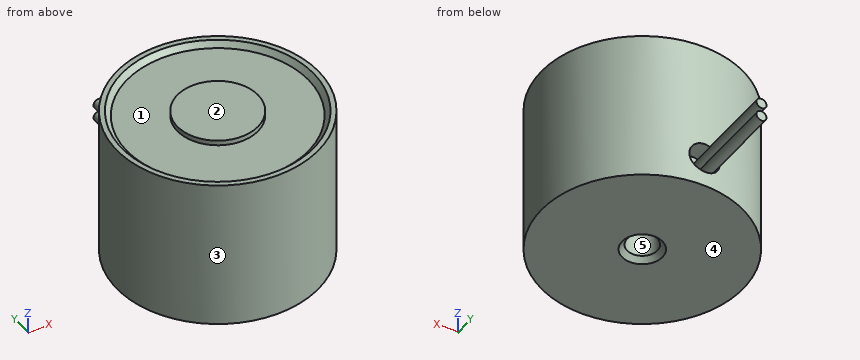
```python
from build123d import *

# Parameters (mm, degrees)
SKETCH_1_R          = 10
EXTRUDE_1_DEPTH     = 15
SKETCH_2_R          = 9
SKETCH_2_R_2        = 4
CUT_EXTRUDE_2_DEPTH = 0.5
CHAMFER_1_SIZE      = 0.5
SKETCH_3_R          = 1.5
CUT_EXTRUDE_3_DEPTH = 5
CHAMFER_2_SIZE      = 0.5
SKETCH_4_R          = 1.5
CUT_EXTRUDE_4_DEPTH = 7
SKETCH_5_R          = 0.5
EXTRUDE_2_DEPTH     = 10


with BuildPart() as part:
    # 草图1 → 凸台-拉伸1 (new body)
    with BuildSketch(Plane.XY):
        Circle(SKETCH_1_R)
    extrude(amount=EXTRUDE_1_DEPTH)

    # 草图2 → 切除-拉伸2 (cut)
    with BuildSketch(Plane.XY.offset(15)):
        Circle(SKETCH_2_R)
        Circle(SKETCH_2_R_2, mode=Mode.SUBTRACT)
    extrude(amount=-CUT_EXTRUDE_2_DEPTH, mode=Mode.SUBTRACT)

    # 倒角1
    chamfer_1_edges = [part.edges().sort_by_distance(p)[0] for p in [
        (-9, 0, 15),
    ]]
    chamfer(chamfer_1_edges, length=CHAMFER_1_SIZE - 0.0001)  # a hair under: the kernel refuses the full size

    # 草图3 → 切除-拉伸3 (cut)
    with BuildSketch(Plane(origin=(0, 0, 0), x_dir=(-1, 0, 0), z_dir=(0, 0, -1))):
        Circle(SKETCH_3_R)
    extrude(amount=-CUT_EXTRUDE_3_DEPTH, mode=Mode.SUBTRACT)

    # 倒角2
    chamfer_2_edges = [part.edges().sort_by_distance(p)[0] for p in [
        (1.5, 0, 0),
    ]]
    chamfer(chamfer_2_edges, length=CHAMFER_2_SIZE)

    # 草图4 → 切除-拉伸4 (cut)
    with BuildSketch(Plane(origin=(0, 8, 0), x_dir=(1, 0, 0), z_dir=(0, 1, 0))):
        with Locations(Location((0, -3, 0), (0, 0, 90))):
            Circle(SKETCH_4_R)
    extrude(amount=CUT_EXTRUDE_4_DEPTH, mode=Mode.SUBTRACT)

    # 草图5 → 凸台-拉伸2 (add)
    with BuildSketch(Plane(origin=(0, 8, 0), x_dir=(1, 0, 0), z_dir=(0, 1, 0))):
        with Locations(Location((-0.6, -2.325227292, 0), (0, 0, 270))):
            Circle(SKETCH_5_R)
        with Locations(Location((-0.6, -3.674772708, 0), (0, 0, 270))):
            Circle(SKETCH_5_R)
    extrude(amount=EXTRUDE_2_DEPTH)


solid = part.part
```
Input: part model. Units: mm. Frame: model coordinates. Face numbers are marked on the shaded views. A direction names the side the tool comes from. Round coordinates to 2 decimals unless told otherwise and drop trailing zeros. Loops run counter-clockwise (first coordinate to the right, second up) from the corner with the lowest first, then second, coordinate; pieces in that order, holes last. Notation, with made-up numbers: (27.25, 60) -> (84.25, 60) arc R15 cw to (84.25, 80) -> close; hole circle Ø7 at (-28.5, -34.5). An arc over 180 degrees is marked (long way). Use one line per item in the form item = value. Start each with the question number.
Item 1: Contact query for flat-ended pins moving along their axis: pin 1 Ø1 at (x, y) = (7, 4) entering from +Z; pin 2 Ø1.5 at (y, z) = (12, 9) entering from -X; pin 3 Ø2 at (x, z) = (7, 8.5) entering from +Y; pin 4 Ø2 at (y, z) = (13, 2) entering from +X. Output: stop coordinate, or through.
Item 2: Section query B-B on y = 14. Return the cut outline in (x, z), then the cut area to 3 significant figures.
Item 3: Section query A-A on z = 2.5. Return the cut outline in (x, y).
Item 4: Set-up query: the marked faces 4 and 5. Return all of +Z, -Z, +X, -X, +Y, -Y with unobstructed straight access to the full face (end or side cutting, diameter ignored); none if empty.
Item 5: Mould query, pull axis Y, two halves, no side actions, for the marked faces 1, 2 and 3. Classes: pulls with the +Y half, pulls with the -Y half, needs draft (parallel to the pull), parting line crosses it, or undercut.
Item 6: Material intervals for L1, parallel to Y at x = 0, z = 2.35; L2, parallel to Z at x = 1.75, y = -5.5; L3, parallel to X at y = 9, z = 3, sorted ascending. Write a range as from..to.
Ans:
q1.pin_1 = 14.5
q1.pin_2 = through
q1.pin_3 = 8
q1.pin_4 = -0.1
q2.outline = circle Ø1 at (-0.6, 2.33); circle Ø1 at (-0.6, 3.67)
q2.area = 1.57 mm^2
q3.outline = (-1.41, 8) -> (-1.41, 9.9) arc R10 ccw (long way) to (1.41, 9.9) -> (1.41, 8) -> (-0.13, 8) -> (-0.13, 18) -> (-1.07, 18) -> (-1.07, 8) -> close; hole circle Ø3 at (0, 0)
q4.face_4 = -Z, +X, -X, +Y, -Y
q4.face_5 = -Z
q5.face_1 = undercut
q5.face_2 = needs draft
q5.face_3 = parting line crosses it
q6.L1 = -10..-1.5, 1.5..8
q6.L2 = 0..14.5
q6.L3 = -4.36..-1.5, 1.5..4.36
